Geometry check sheet. Reference: the model listing, model coordinates, mm. Face numbers are marked on the shaded views. Round coordinates to 2 decimals unless told otherwise and drop trailing zeros. Loops run counter-clockwise (first coordinate to the right, second up) from the corner with the lowest first, then second, coordinate; pieces in that order, holes last.
```python
from build123d import *

# Parameters (mm, degrees)
SKETCH1_W           = 54
SKETCH1_H           = 8
BOSS_EXTRUDE1_DEPTH = 12.7
SKETCH3_W           = 1
SKETCH3_H           = 3.243111396
SKETCH3_H_2         = 4.577374163
CUT_EXTRUDE1_DEPTH  = 2
SKETCH4_R           = 2.3
CUT_EXTRUDE2_DEPTH  = 57.047212241
SKETCH5_R           = 0.6
CUT_EXTRUDE3_DEPTH  = 57.047212241
SKETCH6_R           = 1.2
CUT_EXTRUDE4_DEPTH  = 57.047212241
SKETCH12_R          = 0.6
CUT_EXTRUDE6_DEPTH  = 15
SKETCH14_R          = 0.6
CUT_EXTRUDE7_DEPTH  = 6


with BuildPart() as part:
    # Sketch1 → Boss-Extrude1 (new body)
    with BuildSketch(Plane.XY):
        with Locations((27, 4)):
            Rectangle(SKETCH1_W, SKETCH1_H)
    extrude(amount=BOSS_EXTRUDE1_DEPTH)

    # Sketch3 → Cut-Extrude1 (cut)
    with BuildSketch(Plane(origin=(0, 8, 0), x_dir=(1, 0, 0), z_dir=(0, 1, 0))):
        with Locations((42.087715046, -11.078444302)):
            Rectangle(SKETCH3_W, SKETCH3_H)
        with Locations((42.087715046, -2.288687081)):
            Rectangle(SKETCH3_W, SKETCH3_H_2)
    extrude(amount=-CUT_EXTRUDE1_DEPTH, mode=Mode.SUBTRACT)

    # Sketch4 → Cut-Extrude2 (cut, through all)
    with BuildSketch(Plane.XY.offset(12.7)):
        with Locations(Location((42.087715046, 4, 0), (0, 0, 77.444142201))):
            Circle(SKETCH4_R)
    extrude(amount=-CUT_EXTRUDE2_DEPTH, mode=Mode.SUBTRACT)

    # Sketch5 → Cut-Extrude3 (cut, through all)
    with BuildSketch(Plane(origin=(0, 8, 0), x_dir=(1, 0, 0), z_dir=(0, 1, 0))):
        with Locations(Location((52, -10.5, 0), (0, 0, 270))):
            Circle(SKETCH5_R)
        with Locations(Location((20, -10.5, 0), (0, 0, 270))):
            Circle(SKETCH5_R)
    extrude(amount=-CUT_EXTRUDE3_DEPTH, mode=Mode.SUBTRACT)

    # Sketch6 → Cut-Extrude4 (cut, through all)
    with BuildSketch(Plane.XY.offset(12.7)):
        with Locations((4, 4)):
            Circle(SKETCH6_R)
        with Locations((14, 4)):
            Circle(SKETCH6_R)
    extrude(amount=-CUT_EXTRUDE4_DEPTH, mode=Mode.SUBTRACT)

    # Sketch12 → Cut-Extrude6 (cut)
    with BuildSketch(Plane(origin=(25.944559134, 0, 23.885086629), x_dir=(-0.677303634830695, 0, 0.7357035994509805), z_dir=(-0.7357035994509805, 0, -0.677303634830695))):
        with Locations(Location((-22.135860185, 4, 0), (0, 0, 180))):
            Circle(SKETCH12_R)
    extrude(amount=CUT_EXTRUDE6_DEPTH, mode=Mode.SUBTRACT)

    # Sketch14 → Cut-Extrude7 (cut)
    with BuildSketch(Plane(origin=(0, 0, 0), x_dir=(-1, 0, 0), z_dir=(0, 0, -1))):
        with Locations((-44.387715046, 4)):
            Circle(SKETCH14_R)
    extrude(amount=-CUT_EXTRUDE7_DEPTH, mode=Mode.SUBTRACT)


solid = part.part
```
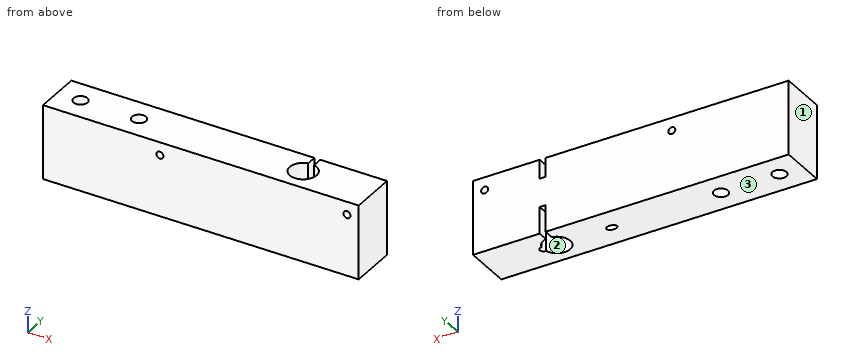
1) Sectioned sample at C-C, the plane y = 4. Record the cut outline in (x, z), then the cut area to 3 significant figures.
Report:
outline: (0, 0) - (2.8, 0) - (2.8, 12.7) - (0, 12.7) - close; (5.2, 0) - (12.8, 0) - (12.8, 12.7) - (5.2, 12.7) - close; (15.2, 0) - (31.8, 0) - (39.79, 7.36) - (39.79, 12.7) - (15.2, 12.7) - close; (33.57, 0) - (39.79, 0) - (39.79, 5.73) - close; (44.39, 6) - (44.99, 6) - (44.99, 0) - (54, 0) - (54, 12.7) - (44.39, 12.7) - close; hole circle Ø1.2 at (20, 10.5); hole circle Ø1.2 at (52, 10.5)
area: 549 mm2
2) Scan lines: line 1 along Y through (x, z) = (14, 1.5); line 2 along X through (y, z) = (7.5, 1.5); line 3 along X through (y, z) = (4.75, 10.5). Record each from-to range of solid material in increasing order.
Report:
line 1: y = 0 to 2.8, 5.2 to 8
line 2: x = 0 to 41.59, 42.59 to 54
line 3: x = 0 to 3.06, 4.94 to 13.06, 14.94 to 19.4, 20.6 to 39.91, 44.26 to 51.4, 52.6 to 54
3) Sectioned sample at B-B, the plane x = 20. Record the cut outline in (y, z).
Report:
outline: (0, 0) - (8, 0) - (8, 9.9) - (0, 9.9) - close; (0, 11.1) - (8, 11.1) - (8, 12.7) - (0, 12.7) - close
4) Sectioned sample at A-A, the plane z = 10.5. Record the cut outline in (x, y) (3 decimals).
Report:
outline: (0, 0) - (19.4, 0) - (19.4, 8) - (0, 8) - close; (20.6, 0) - (51.4, 0) - (51.4, 8) - (42.588, 8) - (42.588, 6.245) arc R2.3 cw (long way) to (41.588, 6.245) - (41.588, 8) - (20.6, 8) - close; (52.6, 0) - (54, 0) - (54, 8) - (52.6, 8) - close; hole circle Ø2.4 at (4, 4); hole circle Ø2.4 at (14, 4)
5) Mould release check, pull along X, two halves, no side actions. Record for the marked faces 1, 2 and 3: +X half, -X half, draft (parallel to the pull), parting line (faces both ways), or undercut.
Report:
face 1: -X half
face 2: undercut
face 3: draft
6) Gauge pin test, flat end, axial feed: pin 1 (0.5 mm diameter, centred on x = 44.5, y = 4, fed in from -Z). Record the tip position at first contact, or that the pin passes through.
Report:
pin 1: stops at z = 6
7) Sectioned sample at D-D, the plane z = 1.25. State how many separate pieces and enclosed holes the cut face has, then the cut area to 3 significant figures.
Report:
separate pieces: 1
enclosed holes: 3
area: 402 mm2
